```python
from build123d import *

# Parameters (mm, degrees)
CROQUIS1_R                = 3.1
SALIENTE_EXTRUIR1_DEPTH   = 6
SALIENTE_EXTRUIR1_2_DEPTH = 6
CROQUIS3_W                = 60
CROQUIS3_H                = 6
SALIENTE_EXTRUIR2_DEPTH   = 16.24
CROQUIS4_W                = 60
CROQUIS4_H                = 112
SALIENTE_EXTRUIR3_DEPTH   = 6
REDONDEO1_R               = 10
CROQUIS5_R                = 3.1
CORTAR_EXTRUIR1_DEPTH     = 264.693121755


with BuildPart() as part:
    # Croquis1 → Saliente-Extruir1 (new body)
    with BuildSketch(Plane.XY):
        with BuildLine():
            Line((51.893497848, -217.1), (111.893497848, -217.1))
            Line((111.893497848, -217.1), (111.893497848, -227.1))
            ThreePointArc((111.893497848, -227.1), (108.96456566, -234.171067812), (101.893497848, -237.1))
            Line((101.893497848, -237.1), (61.893497848, -237.1))
            ThreePointArc((61.893497848, -237.1), (54.822430037, -234.171067812), (51.893497848, -227.1))
            Line((51.893497848, -227.1), (51.893497848, -217.1))
        make_face()
        with Locations(Location((59.893497848, -229.1, 0), (0, 0, 180))):
            Circle(CROQUIS1_R, mode=Mode.SUBTRACT)
        with Locations((103.893497848, -229.1)):
            Circle(CROQUIS1_R, mode=Mode.SUBTRACT)
    extrude(amount=SALIENTE_EXTRUIR1_DEPTH)



with BuildPart() as body_2:
    # Croquis1 → Saliente-Extruir1 2 (new body)
    with BuildSketch(Plane.XY):
        with BuildLine():
            Line((61.893497848, -97.1), (101.893497848, -97.1))
            ThreePointArc((101.893497848, -97.1), (108.96456566, -100.028932188), (111.893497848, -107.1))
            Line((111.893497848, -107.1), (111.893497848, -117.1))
            Line((111.893497848, -117.1), (51.893497848, -117.1))
            Line((51.893497848, -117.1), (51.893497848, -107.1))
            ThreePointArc((51.893497848, -107.1), (54.822430037, -100.028932188), (61.893497848, -97.1))
        make_face()
        with Locations((59.893497848, -105.1)):
            Circle(CROQUIS1_R, mode=Mode.SUBTRACT)
        with Locations(Location((103.893497848, -105.1, 0), (0, 0, 180))):
            Circle(CROQUIS1_R, mode=Mode.SUBTRACT)
    extrude(amount=SALIENTE_EXTRUIR1_2_DEPTH)


with BuildPart() as part_1:
    add(part.part)

    add(body_2.part)  # Saliente-Extruir2 merges body 2
    # Croquis3 → Saliente-Extruir2 (add)
    with BuildSketch(Plane.XY.offset(6)):
        with Locations((81.893497848, -220.1)):
            Rectangle(CROQUIS3_W, CROQUIS3_H)
        with Locations((81.893497848, -114.1)):
            Rectangle(CROQUIS3_W, CROQUIS3_H)
    extrude(amount=SALIENTE_EXTRUIR2_DEPTH)

    # Croquis4 → Saliente-Extruir3 (add)
    with BuildSketch(Plane.XY.offset(22.24)):
        with Locations((81.893497848, -167.1)):
            Rectangle(CROQUIS4_W, CROQUIS4_H)
    extrude(amount=SALIENTE_EXTRUIR3_DEPTH)

    # Redondeo1
    redondeo1_edges = [part_1.edges().sort_by_distance(p)[0] for p in [
        (81.893497848, -217.1, 22.24),
        (81.893497848, -223.1, 28.24),
        (81.893497848, -111.1, 28.24),
        (81.893497848, -117.1, 22.24),
    ]]
    fillet(redondeo1_edges, radius=REDONDEO1_R)

    # Croquis5 → Cortar-Extruir1 (cut, through all)
    with BuildSketch(Plane.XY.offset(28.24)):
        with Locations((105.893497848, -143.1)):
            Circle(CROQUIS5_R)
        with Locations((105.893497848, -191.1)):
            Circle(CROQUIS5_R)
        with Locations((57.893497848, -191.1)):
            Circle(CROQUIS5_R)
        with Locations((57.893497848, -143.1)):
            Circle(CROQUIS5_R)
    extrude(amount=-CORTAR_EXTRUIR1_DEPTH, mode=Mode.SUBTRACT)


solid = part_1.part
```
Could you check a few things on this model? Use its own coordinates, in mm. A direction names the side the tool comes from. Coordinates: 2 decimals unless noted, no trailing zeros. Write each loop counter-clockwise with the first axis right and the second up, starting at its lowest first coordinate (ties: lowest second). Pieces come first, ordered by that corner, then holes. Notation, with made-up numbers: (-37.75, -13.75) -> (-1.75, -13.75) arc R34 ccw to (-1.75, 17.25) -> close; hole circle Ø7 at (15, 71.25). An arc over 180 degrees is marked (long way). One line per question, with ' | ' between items. Start each with the question number.
1. If we section it at A-A (y = -143.1): Please give me the cut outline in (x, z).
2. If we section it at D-D (z = 26): Please give me the cut outline in (x, y), and give its area (3 significant figures).
3. Please list where these lines run through material, in increasing order: line 1 along X through (y, z) = (-191.1, 24.1); line 2 along Y through (x, z) = (67, 3.5); line 3 along Y through (x, z) = (82.5, 8.5).
4. If we section it at C-C (x = 82.5): Please give me the cut outline in (y, z).
5. Thinking about a two-plate mould opening in Y: for faces 1 (the face through (103.221, -232.126, 2.958)), 2 (the face through (105.221, -194.126, 25.282)), 3 (the face through (82, -104, 6)), 4 (the face through (109.042, -234.093, 2.958)), which applies, pulls with the +Y half, pulls with the -Y half, needs draft (parallel to the pull), parting line crosses it, or undercut?
6. Will these pins go through, and if not, where does the flat tip stop? P1, Ø3.5, axis at x = 81.5, z = 8.5, coming from the -Y side; P2, Ø4, axis at x = 58.5, z = 17, coming from the +Y side; P3, Ø4, axis at x = 88, y = -105.5, coming from the +Z side.
7. If we section it at B-B (z = 2.5): Please give me the cut outline in (x, y).
8. For faces 5 (the face through (81, -167, 22.24)), 6 (the face through (81, -223.1, 12)), 7 (the face through (60.297, -232.174, 2.958)), which set-ups out of +Z, -Z, +X, -X, +Y, -Y let a thin tool reach every point of the face, with its end or its side?
Return value:
1) outline: (51.89, 22.24) -> (54.79, 22.24) -> (54.79, 28.24) -> (51.89, 28.24) -> close; (60.99, 22.24) -> (102.79, 22.24) -> (102.79, 28.24) -> (60.99, 28.24) -> close; (108.99, 22.24) -> (111.89, 22.24) -> (111.89, 28.24) -> (108.99, 28.24) -> close
2) outline: (51.89, -219.41) -> (111.89, -219.41) -> (111.89, -114.79) -> (51.89, -114.79) -> close; hole circle Ø6.2 at (57.89, -191.1); hole circle Ø6.2 at (57.89, -143.1); hole circle Ø6.2 at (105.89, -191.1); hole circle Ø6.2 at (105.89, -143.1) | area: 6,160 mm²
3) line 1: x = 51.89 to 54.79, 60.99 to 102.79, 108.99 to 111.89 | line 2: y = -237.1 to -217.1, -117.1 to -97.1 | line 3: y = -223.1 to -217.1, -117.1 to -111.1
4) outline: (-237.1, 0) -> (-217.1, 0) -> (-217.1, 12.24) arc R10 cw to (-207.1, 22.24) -> (-127.1, 22.24) arc R10 cw to (-117.1, 12.24) -> (-117.1, 0) -> (-97.1, 0) -> (-97.1, 6) -> (-111.1, 6) -> (-111.1, 18.24) arc R10 ccw to (-121.1, 28.24) -> (-213.1, 28.24) arc R10 ccw to (-223.1, 18.24) -> (-223.1, 6) -> (-237.1, 6) -> close
5) face 1: undercut | face 2: undercut | face 3: needs draft | face 4: pulls with the -Y half
6) P1: stops at y = -223.1 | P2: stops at y = -111.1 | P3: stops at z = 6
7) outline: (51.89, -227.1) arc R10 ccw to (61.89, -237.1) -> (101.89, -237.1) arc R10 ccw to (111.89, -227.1) -> (111.89, -217.1) -> (51.89, -217.1) -> close; (51.89, -117.1) -> (111.89, -117.1) -> (111.89, -107.1) arc R10 ccw to (101.89, -97.1) -> (61.89, -97.1) arc R10 ccw to (51.89, -107.1) -> close; hole circle Ø6.2 at (59.89, -229.1); hole circle Ø6.2 at (59.89, -105.1); hole circle Ø6.2 at (103.89, -229.1); hole circle Ø6.2 at (103.89, -105.1)
8) face 5: -Z, +X, -X | face 6: +Z, +X, -X, -Y | face 7: +Z, -Z
